```python
from build123d import *

# Parameters (mm, degrees)
F0_R     = 57.15
F0_R_2   = 1.5875
F0_R_3   = 32.8090175067
F1_DEPTH = 3
F0_R_4   = 30.8090175067
F2_DEPTH = 60
F3_DEPTH = 55
F5_DEPTH = 40.5


with BuildPart() as f1:
    # F0 (on Top) → F1 (new body)
    with BuildSketch(Plane.XY):
        Circle(F0_R)
        with Locations((-35.9840175067, 0)):
            Circle(F0_R_2, mode=Mode.SUBTRACT)
        Circle(F0_R_3, mode=Mode.SUBTRACT)
        with Locations((35.9840175067, 0)):
            Circle(F0_R_2, mode=Mode.SUBTRACT)
    extrude(amount=F1_DEPTH)

    # F0 (on Top) → F2 (join)
    with BuildSketch(Plane.XY):
        Circle(F0_R_3)
        Circle(F0_R_4, mode=Mode.SUBTRACT)
        Circle(F0_R_4)
    extrude(amount=F2_DEPTH)

    # F0 (on Top) → F3 (cut)
    with BuildSketch(Plane.XY):
        Circle(F0_R_4)
    extrude(amount=F3_DEPTH, mode=Mode.SUBTRACT)

    # F4 (on Front) → F5 (cut, symmetric)
    with BuildSketch(Plane.XZ):
        with BuildLine():
            Line((32.8090175067, 60), (-32.8090175067, 60))
            ThreePointArc((-32.8090175067, 60), (0, 55.4277625628), (32.8090175067, 60))
        make_face()
    extrude(amount=F5_DEPTH, both=True, mode=Mode.SUBTRACT)


solid = f1.part
```
Here's how the part is built. I have some questions about the finished solid (model axes, mm). A direction names the side the tool comes from. Round coordinates to 2 decimals unless told otherwise and drop trailing zeros. Loops run counter-clockwise (first coordinate to the right, second up) from the corner with the lowest first, then second, coordinate; pieces in that order, holes last. Notation, with made-up numbers: (27, 83) -> (73, 83) arc R13 ccw to (73, 102) -> close; hole circle Ø1 at (-24, -18.75). An arc over 180 degrees is marked (long way). Answer as CSV lines item,"result".
1. Which directions (+Z, -Z, +X, -X, +Y, -Y) give clear straight access to the entire face, cutting with the end or side of a thin tool? Please do faces 1 (the face through (34.4, 0.1, 1.5)), 2 (the face through (25, -25, 3)), 3 (the face through (0, 0, 55)).
Final values:
face 1,"+Z, -Z"
face 2,"+Z"
face 3,"-Z"
2. If we section it at D-D on y = 16: Please give me the cut outline in (x, z), plus the area to 3 significant figures.
Final values:
outline,"(-54.86, 0) -> (-26.33, 0) -> (-26.33, 55) -> (26.33, 55) -> (26.33, 0) -> (54.86, 0) -> (54.86, 3) -> (28.64, 3) -> (28.64, 58.9) arc R120 cw to (-28.64, 58.9) -> (-28.64, 3) -> (-54.86, 3) -> close"
area,"502 mm^2"
3. For pin 1 (6 mm diameter, centred on x = -30, y = 25.5, fed in from -Z); pin 2 (12 mm diameter, centred on x = 40, z = 6.5, fed in from -Y); pin 3 (6 mm diameter, centred on x = -20.5, z = 14.5, fed in from +Y); pin 4 (12 mm diameter, centred on x = 34, z = 27, fed in from -Y), each with a flat end and sliding along its axis, tell me the tip position at first contact or that it passes through.
Final values:
pin 1,"stops at z = 0"
pin 2,"stops at y = -45.08"
pin 3,"stops at y = 27.75"
pin 4,"stops at y = -17.1"
4. If we section it at C-C on z = 53: Please give me the cut outline in (x, y), plus the area to 3 significant figures.
Final values:
outline,"circle Ø65.62 at (0, 0); hole circle Ø61.62 at (0, 0)"
area,"400 mm^2"
5. Thinking about a two-plate mould opening in Y: for faces 4 (the face through (-0.47, -0.46, 55.43)), 5 (the face through (-4.27, 32.53, 31.1)), 6 (the face through (29.386, 9.254, 27.115)), which applies, released by +Y, released by -Y, zero draft, split by the parting line, or undercut?
Final values:
face 4,"zero draft"
face 5,"split by the parting line"
face 6,"undercut"
6. If we section it at B-B on x = 0: Please give me the cut outline in (y, z).
Final values:
outline,"(-57.15, 0) -> (-30.81, 0) -> (-30.81, 55) -> (30.81, 55) -> (30.81, 0) -> (57.15, 0) -> (57.15, 3) -> (32.81, 3) -> (32.81, 55.43) -> (-32.81, 55.43) -> (-32.81, 3) -> (-57.15, 3) -> close"
7. If I drill on L1, parallel to X at y = -1, z = 17.5; L2, parallel to Z at x = -35, y = -27; L3, parallel to Y at x = 17, z = 42, over which ranges is the centre line in solid material (lowest first)?
Final values:
L1,"x = -32.79 to -30.79, 30.79 to 32.79"
L2,"z = 0 to 3"
L3,"y = -28.06 to -25.69, 25.69 to 28.06"
8. If we section it at A-A on y = 0: Please give me the cut outline in (x, z).
Final values:
outline,"(-57.15, 0) -> (-37.57, 0) -> (-37.57, 3) -> (-57.15, 3) -> close; (-34.4, 0) -> (-30.81, 0) -> (-30.81, 55) -> (30.81, 55) -> (30.81, 0) -> (34.4, 0) -> (34.4, 3) -> (32.81, 3) -> (32.81, 60) arc R120 cw to (-32.81, 60) -> (-32.81, 3) -> (-34.4, 3) -> close; (37.57, 0) -> (57.15, 0) -> (57.15, 3) -> (37.57, 3) -> close"
